from build123d import *

# Parameters (mm, degrees)
BOSS_EXTRU_1_DEPTH           = 12.7
ESQUISSE2_R                  = 3.175
ENL_V_MAT_EXTRU_1_DEPTH      = 21.875
ENL_V_MAT_EXTRU_1_DEPTH_BACK = 9.175
CONG_2_R                     = 1
ENL_V_MAT_EXTRU_2_REACH      = 48.05
ESQUISSE3_R                  = 2.5


with BuildPart() as part:
    # Esquisse1 → Boss.-Extru.1 (new body)
    with BuildSketch(Plane.XY):
        with BuildLine():
            Line((0, 41.05), (0, 46.05))
            Line((0, 46.05), (-14.525, 46.05))
            Line((-14.525, 46.05), (-14.525, 0))
            Line((-14.525, 0), (-6.35, 0))
            Line((-6.35, 0), (-6.35, 17))
            Line((-6.35, 17), (0, 17))
            Line((0, 17), (0, 22))
            Line((0, 22), (-8.525, 22))
            ThreePointArc((-8.525, 22), (-10.232106781, 21.292893219), (-9.525, 23))
            Line((-9.525, 23), (-9.525, 40.05))
            ThreePointArc((-9.525, 40.05), (-10.232106781, 41.757106781), (-8.525, 41.05))
            Line((-8.525, 41.05), (0, 41.05))
        make_face()
        with BuildLine():
            Line((14.525, 0), (14.525, 46.05))
            Line((14.525, 46.05), (0, 46.05))
            Line((0, 46.05), (0, 41.05))
            Line((0, 41.05), (8.525, 41.05))
            ThreePointArc((8.525, 41.05), (9.525, 42.05), (10.525, 41.05))
            ThreePointArc((10.525, 41.05), (10.232106781, 40.342893219), (9.525, 40.05))
            Line((9.525, 40.05), (9.525, 23))
            ThreePointArc((9.525, 23), (10.232106781, 22.707106781), (10.525, 22))
            ThreePointArc((10.525, 22), (9.525, 21), (8.525, 22))
            Line((8.525, 22), (0, 22))
            Line((0, 22), (0, 17))
            Line((0, 17), (6.35, 17))
            Line((6.35, 17), (6.35, 0))
            Line((6.35, 0), (14.525, 0))
        make_face()
    extrude(amount=BOSS_EXTRU_1_DEPTH)

    # Esquisse2 → Enlèv. mat.-Extru.1 (cut, two sides)
    with BuildSketch(Plane(origin=(-6.35, 0, 0), x_dir=(0, 0, -1), z_dir=(1, 0, 0))) as enl_v_mat_extru_1_sk:
        with Locations((-6.35, 6.35)):
            Circle(ESQUISSE2_R)
    extrude(amount=ENL_V_MAT_EXTRU_1_DEPTH, mode=Mode.SUBTRACT)
    extrude(enl_v_mat_extru_1_sk.sketch, amount=-ENL_V_MAT_EXTRU_1_DEPTH_BACK, mode=Mode.SUBTRACT)

    # Congé2
    cong_2_edges = [part.edges().sort_by_distance(p)[0] for p in [
        (14.525, 0, 6.35),
        (6.35, 0, 6.35),
        (6.35, 17, 6.35),
        (-6.35, 17, 6.35),
        (-6.35, 0, 6.35),
        (-14.525, 0, 6.35),
        (-14.525, 46.05, 6.35),
        (14.525, 46.05, 6.35),
    ]]
    fillet(cong_2_edges, radius=CONG_2_R)

    # Esquisse3 → Enlèv. mat.-Extru.2 (cut, up to next)
    with BuildSketch(Plane(origin=(0, 46.05, 0), x_dir=(1, 0, 0), z_dir=(0, 1, 0)), mode=Mode.PRIVATE) as enl_v_mat_extru_2_sk1:
        with Locations((0, -6.35)):
            Circle(ESQUISSE3_R)
    enl_v_mat_extru_2_tool1 = extrude(enl_v_mat_extru_2_sk1.sketch, amount=-ENL_V_MAT_EXTRU_2_REACH, mode=Mode.PRIVATE) & part.part
    add(enl_v_mat_extru_2_tool1.solids().sort_by_distance((0, 46.05, 6.35))[0], mode=Mode.SUBTRACT)


solid = part.part
Here's how the part is built. I have some questions about the finished solid (model axes, mm). A direction names the side the tool comes from. Give positions to 0.01 mm unless a question says otherwise; leave off trailing zeros. Order: outer loops, then holes, each group sorted by start corner. A loop starts at its lowest first (then second) coordinate and runs counter-clockwise, first axis right, second up. Notation, with made-up numbers: M -5,-33.5 L 28,-33.5 A22 cw 28,5.5 Z; hole C 77.25,20 d10. An arc over 180 degrees is marked long. Answer as a JSON object with one key per item and string values. Group by question number.
1) Suppose I cut it at A-A, the plane x = 0. Write out the boundary of the cut face in (y, z), plus the area to 3 significant figures.
2) Suppose I cut it at D-D, the plane y = 6.35. Write out the boundary of the cut face in (x, z) (3 decimals).
3) Suppose I cut it at B-B, the plane y = 31. Write out the boundary of the cut face in (x, z) (3 decimals).
4) I'm going to push flat-ended pins straight in: pin 1 Ø12 at (x, y) = (-8.5, 30) entering from +Z; pin 2 Ø6.5 at (x, z) = (0, 6.35) entering from -Y. Where does each tip first touch, or does it pass through?
5) We'd pull the mould along X, two halves only. Please class faces 1 (the cylindrical face through (10.4, 9, 4.6)), 2 (the cylindrical face through (-6.065, 16.699, 6.439)), 3 (the cylindrical face through (-14.24, 45.75, 6.44)): pulls with the +X half, pulls with the -X half, needs draft (parallel to the pull), parting line crosses it, or undercut.
6) On a 3-axis mill with a long thin cutter (end or side, diameter ignored), from which of +Z, -Z, +X, -X, +Y, -Y can I reach the whole of each face in a straight line? I mean faces 4 (the cylindrical face through (14.224, 45.765, 6.439)), 5 (the flat face through (10, 0, 6)), 6 (the flat face through (9.525, 32, 6)), 7 (the cylindrical face through (-1.984, 43.585, 7.871)), 8 (the cylindrical face through (-6.651, 0.285, 6.439)). Say none if no direction works.
7) Please list where these lines run through material, in increasing order: L1, parallel to Y at x = 11.75, z = 6.25; L2, parallel to X at y = 37, z = 8.5 (3 decimals); L3, parallel to X at y = 13.5, z = 8.5 (3 decimals). Write a range as [from, to].
8) Suppose I cut it at C-C, the plane z = 10.5. Write out the boundary of the cut face in (x, y) (3 decimals), plus the area to 3 significant figures.
Results found:
{
 "1": {"outline": "M 17,0 L 22,0 L 22,12.7 L 17,12.7 Z; M 41.05,0 L 46.05,0 L 46.05,3.85 L 41.05,3.85 Z; M 41.05,8.85 L 46.05,8.85 L 46.05,12.7 L 41.05,12.7 Z", "area": "102 mm²"},
 "2": {"outline": "M -14.525,0 L -6.35,0 L -6.35,3.175 L -14.525,3.175 Z; M -14.525,9.525 L -6.35,9.525 L -6.35,12.7 L -14.525,12.7 Z; M 6.35,0 L 14.525,0 L 14.525,3.175 L 6.35,3.175 Z; M 6.35,9.525 L 14.525,9.525 L 14.525,12.7 L 6.35,12.7 Z"},
 "3": {"outline": "M -14.525,0 L -9.525,0 L -9.525,12.7 L -14.525,12.7 Z; M 9.525,0 L 14.525,0 L 14.525,12.7 L 9.525,12.7 Z"},
 "4": {"pin 1": "z = 12.7", "pin 2": "y = 17"},
 "5": {"face 1": "needs draft", "face 2": "undercut", "face 3": "pulls with the -X half"},
 "6": {"face 4": "+Z, -Z, +X, +Y", "face 5": "+Z, -Z, +X, -X, -Y", "face 6": "+Z, -Z", "face 7": "+Y", "face 8": "+Z, -Z, -Y"},
 "7": {"L1": "[0, 3.18], [9.52, 46.05]", "L2": "[-14.525, -9.525], [9.525, 14.525]", "L3": "[-14.525, -6.35], [6.35, 14.525]"},
 "8": {"outline": "M -14.525,1 A1 ccw -13.525,0 L -7.35,0 A1 ccw -6.35,1 L -6.35,16 A1 cw -5.35,17 L 5.35,17 A1 cw 6.35,16 L 6.35,1 A1 ccw 7.35,0 L 13.525,0 A1 ccw 14.525,1 L 14.525,45.05 A1 ccw 13.525,46.05 L -13.525,46.05 A1 ccw -14.525,45.05 Z; hole M -9.525,23 A1 ccw long -8.525,22 L 8.525,22 A1 ccw long 9.525,23 L 9.525,40.05 A1 ccw long 8.525,41.05 L -8.525,41.05 A1 ccw long -9.525,40.05 Z", "area": "749 mm²"}
}
